from build123d import *

# Parameters (mm, degrees)
F1_DEPTH = 1828.8
F3_D     = 12.7
F5_D     = 9.525
F6_ANGLE = 180
F9_D     = 7.9375


# Not quite as in the source:
# - a length typed as a fraction of an inch, garbled in the dataset ("3 / 203.2 mm" for 3/8 in), is restored
# - a feature names something its author has since deleted; it is built from what else it names


with BuildPart() as f1:
    # F0 (on Front) → F1 (new body)
    with BuildSketch(Plane.XZ):
        Polygon((-59.9026924796, 82.7025878191), (-59.9026924796, 6.5025878191), (16.2973075204, 6.5025878191), (16.2973075204, 11.2650878191), (-55.1401924796, 11.2650878191), (-55.1401924796, 82.7025878191), align=None)
    extrude(amount=F1_DEPTH)

    # F3 (through all)
    with Locations(Plane.YZ.offset(-55.1401924796)):
        with Locations((-203.2, 63.6525878191), (-1625.6, 63.6525878191)):
            Hole(F3_D / 2)

    # F5 (through all)
    with Locations(Plane(origin=(0, 0, 0), x_dir=(1, 0, 0), z_dir=(0, 0, -1))):
        with Locations((-28.1526924796, 1371.6), (-2.7526924796, 1676.4), (-2.7526924796, 1066.8), (-28.1526924796, 762), (-2.7526924796, 457.2), (-28.1526924796, 152.4)):
            Hole(F5_D / 2)


with BuildPart() as f1_1:
    # F6: moved
    add(f1.part.rotate(Axis((-19.4214424796, -1828.8, 11.2650878191), (-1, 0, 0)), F6_ANGLE))


with BuildPart() as f1_2:
    # F7: moved
    add(f1_1.part.moved(Location((0, 1828.8, 0))))

    # F9 (through all)
    with Locations(Plane.YZ.offset(-55.1401924796)):
        with Locations((-152.4, -1.4349121809), (-304.8, -1.4349121809), (-457.2, -1.4349121809), (-609.6, -1.4349121809), (-762, -1.4349121809), (-914.4, -1.4349121809), (-1066.8, -1.4349121809), (-1219.2, -1.4349121809), (-1371.6, -1.4349121809), (-1524, -1.4349121809), (-1676.4, -1.4349121809)):
            Hole(F9_D / 2)


solid = f1_2.part
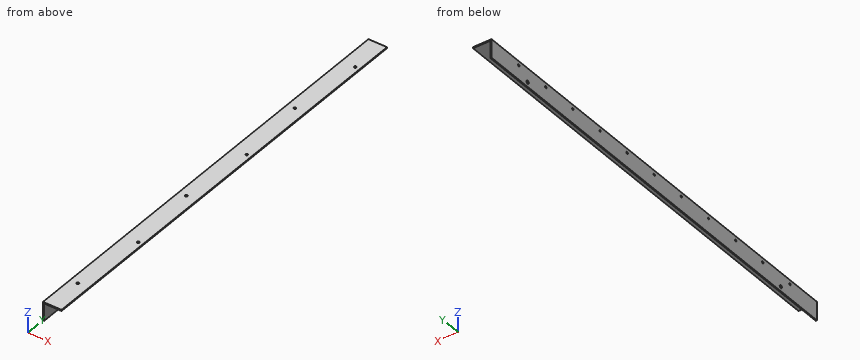
Geometry check sheet. Reference: the model listing, model coordinates, mm. Round coordinates to 2 decimals unless told otherwise and drop trailing zeros. Write each loop counter-clockwise with the first axis right and the second up, starting at its lowest first coordinate (ties: lowest second). Pieces come first, ordered by that corner, then holes. Notation, with made-up numbers: (-13, -4.75) -> (44, -4.75) arc R23 ccw to (44, 21.25) -> close; hole circle Ø11 at (-34, 75). An arc over 180 degrees is marked (long way). One line per item, written item: value. Start each with the question number.
(1) Scan lines: line 1 (Z direction, x = -57.2, y = -762); line 2 (Z direction, x = -56, y = -203); line 3 (X direction, y = -1178, z = -44). Record each from-to range of solid material in increasing order. Write a range as [from, to].
(2) Cross-section at A-A, the plane y = -1718. Record the cut outline in (x, z).
(3) Go/stop test with flat-tipped pins: pin 1 Ø6 at (x, y) = (-26, -652) entering from -Z; pin 2 Ø9 at (y, z) = (-1371.6, -1.43) entering from +X. Record where each tip stops, or that it passes through.
Answer:
1. line 1: [-60.17, -5.4], [2.53, 16.03]
1. line 2: [-60.17, -47.47], [-34.78, 16.03]
1. line 3: [-59.9, -55.14]
2. outline: (-59.9, -60.17) -> (-55.14, -60.17) -> (-55.14, 11.27) -> (16.3, 11.27) -> (16.3, 16.03) -> (-59.9, 16.03) -> close
3. pin 1: z = 11.27
3. pin 2: x = -55.14
